Geometry check sheet. Reference: drawing and pictorial views, mm from the part's lowest x, y, z. Give positions to 0.01 mm unless a question says otherwise; leave off trailing zeros. Order: outer loops, then holes, each group sorted by start corner. A loop starts at its lowest first (then second) coordinate and runs counter-clockwise, first axis right, second up. Notation, with made-up numbers: M 81,27.25 L 113,27.25 A30 ccw 113,61.25 Z; hole C 47.25,16.25 d11. An arc over 180 degrees is marked long. Answer as CSV lines item,"result".
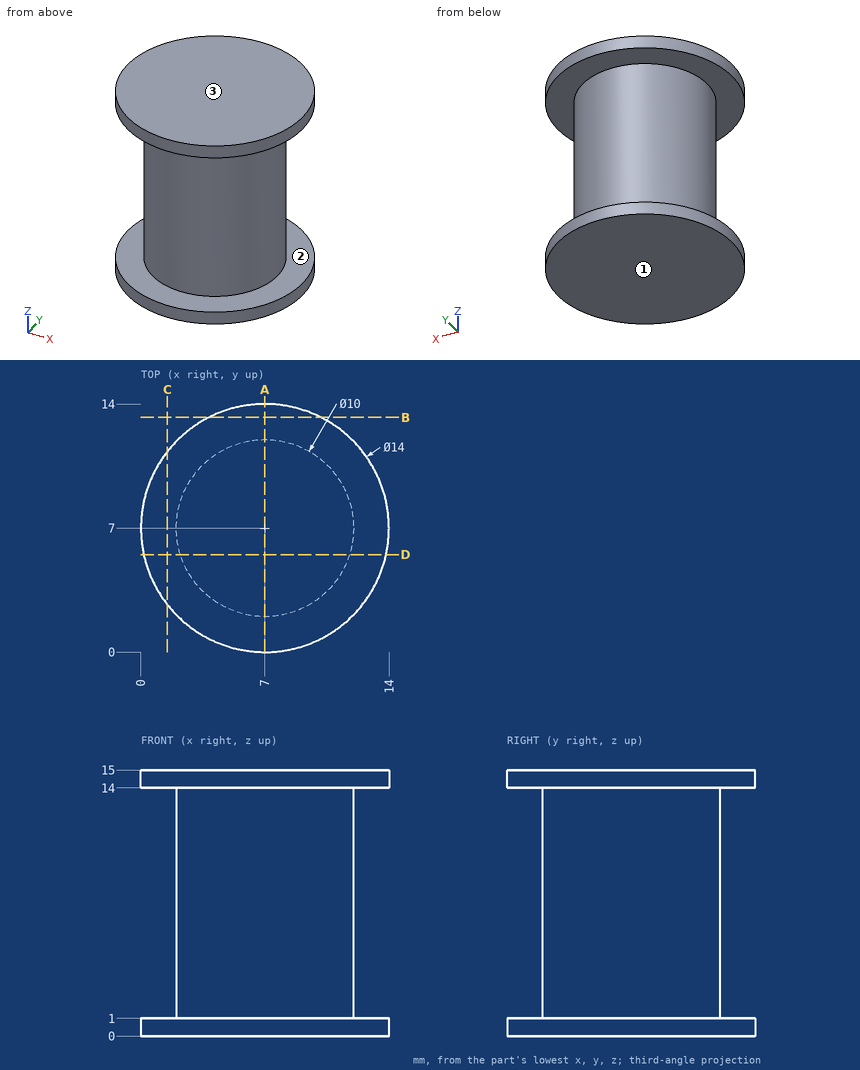
(1) Section check C-C on x = 1.5. Enter the section's corners in (y, z), then the cut area to 3 significant figures.
The answers:
outline,"M 2.67,0 L 11.33,0 L 11.33,1 L 2.67,1 Z; M 2.67,14 L 11.33,14 L 11.33,15 L 2.67,15 Z"
area,"17.3 mm2"
(2) Section check A-A on x = 7. Enter the section's corners in (y, z).
The answers:
outline,"M 0,0 L 14,0 L 14,1 L 12,1 L 12,14 L 14,14 L 14,15 L 0,15 L 0,14 L 2,14 L 2,1 L 0,1 Z"
(3) Section check B-B on y = 13.25. Enter the section's corners in (x, z).
The answers:
outline,"M 3.85,0 L 10.15,0 L 10.15,1 L 3.85,1 Z; M 3.85,14 L 10.15,14 L 10.15,15 L 3.85,15 Z"
(4) Draft check along Z on the marked faces 1, 2 and 3. Enter one of: +Z half, -Z half, draft (parallel to the pull), parting line (faces both ways), or undercut.
The answers:
face 1,"-Z half"
face 2,"undercut"
face 3,"+Z half"
(5) Section check D-D on y = 5.5. Enter the section's corners in (x, z).
The answers:
outline,"M 0.16,0 L 13.84,0 L 13.84,1 L 11.77,1 L 11.77,14 L 13.84,14 L 13.84,15 L 0.16,15 L 0.16,14 L 2.23,14 L 2.23,1 L 0.16,1 Z"
(6) Gauge pin test, flat ends, axial feed: P1, Ø1, axis at x = 5, z = 7.5, coming from the -Y side; P2, Ø2, axis at y = 2, z = 1.5, coming from the +X side; P3, Ø3, axis at x = 4.5, z = 4, coming from the +Y side. Record the tip position at first contact, or that the pin passes through.
The answers:
P1,"stops at y = 2.23"
P2,"stops at x = 12.65"
P3,"stops at y = 11.9"
(7) Material ranges on line 1 (Z direction, x = 12, y = 8.5); line 2 (X direction, y = 8, z = 3.5); line 3 (X direction, y = 5.5, z = 4.5), recorded low to high.
The answers:
line 1,"z = 0 to 1, 14 to 15"
line 2,"x = 2.1 to 11.9"
line 3,"x = 2.23 to 11.77"
